Geometry: final body of the model. Coordinates: model frame, mm. Coordinates: 2 decimals unless noted, no trailing zeros. Order: outer loops, then holes, each group sorted by start corner. A loop starts at its lowest first (then second) coordinate and runs counter-clockwise, first axis right, second up. Notation, with made-up numbers: M 28,33.5 L 69,33.5 A24 cw 69,52.5 Z; hole C 34.5,1 d3. An arc over 180 degrees is marked long. Use CSV: the item, a comma, the result in double quotes. Start each with the question number.
1. First-contact query: P1, Ø0.6, axis at y = -17.5, z = 2, coming from the +X side; P2, Ø1, axis at x = -23, z = 1.5, coming from the +Y side; P3, Ø0.6, axis at y = -26.5, z = 2, coming from the +X side; P4, Ø3.5, axis at x = 10.96, y = 36.97, coming from the -Z side. Flat tips, straight axial feed; report the tip coordinate or a pass-through.
2. Section query B-B on y = 4.5. Return the cut outline in (x, z) (3 decimals).
3. Section query C-C on z = 1.8. State how many separate pieces and enclosed holes the cut face has, and give its area (3 significant figures).
4. Section query A-A on x = 34. Return the cut outline in (y, z) (3 decimals), and give its area (3 significant figures).
5. Pull-direction query (Y, two-part tool) for faces 1 (the flat face through (-14.8, 34.725, 1.565)), 2 (the flat face through (-17, 14, 3.175)), 3 (the flat face through (22.54, 21.01, 1.57)); classes: pulls with the +Y half, pulls with the -Y half, needs draft (parallel to the pull), parting line crosses it, or undercut.
6. Material intervals for line 1 (Y direction, x = -14, z = 2); line 2 (Y direction, x = -15.5, z = 2.4); line 3 (X direction, y = 40, z = 0.35), sorted ascending.
from build123d import *

# Parameters (mm, degrees)
F0_W     = 5.08
F0_H     = 1.836467
F0_H_2   = 1.836468
F0_R     = 1.8415
F0_W_2   = 3.175
F0_H_3   = 1.5875
F1_DEPTH = 3.175


with BuildPart() as f1:
    # F0 (on Top) → F1 (new body)
    with BuildSketch(Plane.XY):
        Polygon((1.5875, -29.071287), (44.449999, -29.079242), (0.005395, 72.529008), (-44.449999, -29.062744), (-1.5875, -29.070698), (-1.5875, -27.483493), (0, -27.483493), (1.5875, -27.483493), align=None)
        with Locations((-35.429051, -26.18307)):
            Rectangle(F0_W, F0_H, mode=Mode.SUBTRACT)
        with Locations((-35.429051, -17.234603)):
            Rectangle(F0_W, F0_H_2, mode=Mode.SUBTRACT)
        with BuildLine():
            ThreePointArc((1.8415, -24.625993), (1.302137, -25.92813), (0, -26.467493))
            ThreePointArc((0, -26.467493), (-1.8415, -24.625993), (0, -22.784493))
            ThreePointArc((0, -22.784493), (1.302137, -23.323855), (1.8415, -24.625993))
        make_face(mode=Mode.SUBTRACT)
        Polygon((-24.382213, 15.910164), (-23.007653, 15.116562), (-24.595153, 12.366931), (-25.969713, 13.160534), align=None, mode=Mode.SUBTRACT)
        with Locations((-21.326735, 12.312996)):
            Circle(F0_R, mode=Mode.SUBTRACT)
        Polygon((1.5875, -21.768493), (0, -21.768493), (-1.5875, -21.768493), (-1.5875, -20.180698), (-30.857051, -20.175266), (-18.039491, 9.116081), (-18.270747, 8.715534), (-19.645818, 9.509431), (-18.058318, 12.259062), (-16.945342, 11.616485), (0.003745, 50.349411), (16.945842, 11.616773), (18.058318, 12.259062), (19.645818, 9.509431), (18.270747, 8.715534), (18.040242, 9.11478), (30.857051, -20.186719), (1.5875, -20.181287), align=None, mode=Mode.SUBTRACT)
        with Locations((35.429051, -26.18307)):
            Rectangle(F0_W, F0_H, mode=Mode.SUBTRACT)
        with Locations((35.429051, -17.234603)):
            Rectangle(F0_W, F0_H_2, mode=Mode.SUBTRACT)
        with Locations((21.326735, 12.312996)):
            Circle(F0_R, mode=Mode.SUBTRACT)
        Polygon((25.969713, 13.160534), (24.595153, 12.366931), (23.007653, 15.116562), (24.382213, 15.910164), align=None, mode=Mode.SUBTRACT)
        Polygon((-12.642652, 34.163247), (-14.017468, 33.369497), (-15.604968, 36.119127), (-14.230152, 36.912878), align=None, mode=Mode.SUBTRACT)
        with Locations((-10.961735, 36.966812)):
            Circle(F0_R, mode=Mode.SUBTRACT)
        Polygon((-6.318502, 37.814497), (-7.693317, 37.020747), (-9.280817, 39.770378), (-7.906002, 40.564128), align=None, mode=Mode.SUBTRACT)
        with Locations((-0.001844, 52.305038)):
            Rectangle(F0_W_2, F0_H_3, mode=Mode.SUBTRACT)
        with Locations((-0.001844, 55.956288)):
            Circle(F0_R, mode=Mode.SUBTRACT)
        with Locations((-0.001844, 59.607538)):
            Rectangle(F0_W_2, F0_H_3, mode=Mode.SUBTRACT)
        with Locations((10.963579, 36.970006)):
            Circle(F0_R, mode=Mode.SUBTRACT)
        Polygon((7.907846, 40.567321), (9.282661, 39.773571), (7.695161, 37.023941), (6.320346, 37.817691), align=None, mode=Mode.SUBTRACT)
        Polygon((14.231996, 36.916071), (15.606812, 36.122321), (14.019312, 33.372691), (12.644496, 34.166441), align=None, mode=Mode.SUBTRACT)
    extrude(amount=F1_DEPTH)


solid = f1.part
Results list:
1,P1,"stops at x = 39.52"
1,P2,"stops at y = 21.1"
1,P3,"stops at x = 43.45"
1,P4,"passes through"
2,outline,"M -29.763,0 L -20.059,0 L -20.059,3.175 L -29.763,3.175 Z; M 20.059,0 L 29.762,0 L 29.762,3.175 L 20.059,3.175 Z"
3,separate pieces,"1"
3,enclosed holes,"19"
3,area,"2,180 mm²"
4,outline,"M -29.077,0 L -27.101,0 L -27.101,3.175 L -29.077,3.175 Z; M -25.265,0 L -18.153,0 L -18.153,3.175 L -25.265,3.175 Z; M -16.316,0 L -5.189,0 L -5.189,3.175 L -16.316,3.175 Z"
4,area,"64.2 mm²"
5,face 1,"undercut"
5,face 2,"needs draft"
5,face 3,"pulls with the +Y half"
6,line 1,"y = -29.07 to -20.18, 18.35 to 33.38, 36.51 to 40.52"
6,line 2,"y = -29.07 to -20.18, 14.92 to 35.94, 36.18 to 37.1"
6,line 3,"x = -14.23 to -8.88, -7.58 to -4.53, 4.53 to 7.58, 8.89 to 14.23"
